Autodesk Inventor part; units mm, degrees
ref_plane "Work Plane1" through (0, 0, 39.4615) normal (0, 0, 1) x (1, 0, 0)
ref_plane "Work Plane2" through (-9.545, 0, 0) normal (1, 0, 0) x (0, 1, 0)
ref_plane "XZ Plane" through (0, 0, 0) normal (0, 1, 0) x (-1, 0, 0)
sketch "Sketch1" plane through (0, 0, 0) normal (0, 1, 0) x (-1, 0, 0)
  circle A0 centre (24.5999, -4.9022) radius 2.2225
  line L0 (26.4238, -3.6322) -> (26.6065, -3.6322)
  circle A1 centre (24.5999, 4.9022) radius 2.2225
  line L1 (26.6196, 9.4615) -> (23.1196, 9.4615)
  line L2 (26.6065, -9.4615) -> (20.6065, -9.4615)
  line L3 (26.4238, -6.1722) -> (26.6065, -6.1722)
  line L4 (23.1196, 9.4615) -> (23.1196, 14.4615)
  line L5 (-26.4238, -3.6322) -> (-26.6065, -3.6322)
  line L6 (-26.4238, -6.1722) -> (-26.6065, -6.1722)
  line L7 (-26.6065, -9.4615) -> (-20.6065, -9.4615)
  circle A2 centre (-24.5999, -4.9022) radius 2.2225
  circle A3 centre (-24.5999, 4.9022) radius 2.2225
  line L8 (-26.6196, 9.4615) -> (-23.1196, 9.4615)
  line L9 (-23.1196, 9.4615) -> (-23.1196, 14.4615)
  line L10 (20.6065, 10.9615) -> (-20.6065, 10.9615)
  line L11 (23.1196, 14.4615) -> (21.9202, 14.4615)
  line L12 (-12.375, 14.4615) -> (-23.1196, 14.4615)
  line L13 (21.9202, 14.4593) -> (21.9202, 39.4593)
  line L14 (21.9202, 14.4593) -> (46.9202, 14.4593) construction
  line L15 (21.9202, 39.4593) -> (-2.8298, 39.4615)
  line L16 (-2.8298, 39.4615) -> (-2.832, 14.4615)
  line L17 (-2.832, 14.4615) -> (-12.375, 14.4615)
  line L18 (-26.6196, 9.4615) -> (-29.5802, 9.4615)
  line L19 (-29.5802, 9.4615) -> (-29.5802, -9.4615)
  line L20 (-29.5802, -9.4615) -> (-26.6065, -9.4615)
  line L21 (26.6196, 9.4615) -> (29.5802, 9.4615)
  line L22 (29.5802, 9.4615) -> (29.5802, -9.4615)
  line L23 (29.5802, -9.4615) -> (26.6065, -9.4615)
  line L24 (-20.6065, -9.4615) -> (-20.6065, 10.9615)
  line L25 (20.6065, -9.4615) -> (20.6065, 10.9615)
  point P0 (-26.4238, 3.6322)
  point P1 (0, 0)
  point P2 (9.5452, 14.4593)
  dimension "d38" = 90
  dimension "d39" = 24.75
  dimension "d41" = 90
  dimension "d43" = 4.9803
  dimension "d45" = 4.9803
extrude "Extrusion1" add sketch "Sketch1" along normal blind 3 contours A0 | A1 | L21 L22 L23 L2 L25 L10 L24 L7 L20 L19 L18 L8 L9 L12 L17 L16 L15 L13 L11 L4 L1 | A2 | A3
ref_plane "Work Plane1" through (0, 0, 39.4615) normal (0, 0, 1) x (1, 0, 0)
sketch "Sketch2" plane through (0, 0, 39.4615) normal (0, 0, 1) x (1, 0, 0)
  circle A0 centre (-9.5452, 25) radius 9.125
  line L0 (-21.9202, 0) -> (2.8298, 0)
  arc A1 (2.8298, 25) -> (-21.9202, 25) centre (-9.5452, 25) ccw
  line L1 (2.8298, 0) -> (2.8298, 25)
  line L2 (-21.9202, 0) -> (-21.9202, 25)
  point P0 (0, 0)
  point P1 (-9.5452, 0)
  dimension "d23" = 18.25
  dimension "d24" = 24.75
  dimension "d25" = 24.75
  dimension "d26" = 25
  dimension "d27" = 25
extrude "Extrusion2" add sketch "Sketch2" along normal blind 3
extrude "Extrusion3" cut sketch "Sketch1" along normal up to next contours A0 | A1 | A2 | A3
sketch "Sketch3" plane through (0, 0, 0) normal (0, -1, 0) x (1, 0, 0)
  circle A0 centre (-24.5999, -4.9022) radius 2.2225
  circle A1 centre (-24.5999, 4.9022) radius 2.2225
  circle A2 centre (24.5999, 4.9022) radius 2.2225
  circle A3 centre (24.5999, -4.9022) radius 2.2225
  line L0 (-29.5802, -9.4615) -> (-20.6065, -9.4615)
  line L1 (-20.6065, -9.4615) -> (-20.6065, 10.9615)
  line L2 (-20.6065, 10.9615) -> (20.6065, 10.9615)
  line L3 (20.6065, 10.9615) -> (20.6065, -9.4615)
  line L4 (20.6065, -9.4615) -> (29.5802, -9.4615)
  line L5 (29.5802, -9.4615) -> (29.5802, 9.4615)
  line L6 (29.5802, 9.4615) -> (23.1196, 9.4615)
  line L7 (23.1196, 9.4615) -> (23.1196, 14.4615)
  line L8 (23.1196, 14.4615) -> (2.832, 14.4615)
  line L9 (2.832, 14.4615) -> (2.8298, 39.4615)
  line L10 (2.8298, 39.4615) -> (-21.9202, 39.4593)
  line L11 (-21.9202, 39.4593) -> (-21.9202, 14.4615)
  line L12 (-21.9202, 14.4615) -> (-23.1196, 14.4615)
  line L13 (-23.1196, 14.4615) -> (-23.1196, 9.4615)
  line L14 (-23.1196, 9.4615) -> (-29.5802, 9.4615)
  line L15 (-29.5802, 9.4615) -> (-29.5802, -9.4615)
  line L16 (-21.9202, 39.4615) -> (2.8298, 39.4615)
  line L17 (2.8298, 39.4615) -> (2.8298, 42.4615)
  line L18 (-21.9202, 42.4615) -> (2.8298, 42.4615)
  line L19 (-21.9202, 39.4615) -> (-21.9202, 42.4615)
  point P0 (0, 0)
extrude "Extrusion4" add sketch "Sketch3" along normal blind 2
sketch "Sketch4" plane through (0, -2, 0) normal (0, -1, 0) x (1, 0, 0)
  circle A0 centre (24.5999, -4.9022) radius 2.2225
  circle A1 centre (24.5999, 4.9022) radius 2.2225
  circle A2 centre (-24.5999, 4.9022) radius 2.2225
  circle A3 centre (-24.5999, -4.9022) radius 2.2225
  line L0 (-29.5802, -9.4615) -> (-20.6065, -9.4615)
  line L1 (-20.6065, -9.4615) -> (-20.6065, 10.9615)
  line L2 (-20.6065, 10.9615) -> (20.6065, 10.9615)
  line L3 (20.6065, 10.9615) -> (20.6065, -9.4615)
  line L4 (20.6065, -9.4615) -> (29.5802, -9.4615)
  line L5 (29.5802, -9.4615) -> (29.5802, 9.4615)
  line L6 (29.5802, 9.4615) -> (23.1196, 9.4615)
  line L7 (23.1196, 9.4615) -> (23.1196, 14.4615)
  line L8 (23.1196, 14.4615) -> (2.832, 14.4615)
  line L9 (2.832, 14.4615) -> (2.8298, 39.4615)
  line L10 (2.8298, 39.4615) -> (-21.9202, 39.4593)
  line L11 (-21.9202, 39.4593) -> (-21.9202, 14.4615)
  line L12 (-21.9202, 14.4615) -> (-23.1196, 14.4615)
  line L13 (-23.1196, 14.4615) -> (-23.1196, 9.4615)
  line L14 (-23.1196, 9.4615) -> (-29.5802, 9.4615)
  line L15 (-29.5802, 9.4615) -> (-29.5802, -9.4615)
  line L16 (2.832, 14.4615) -> (23.1196, 14.4615)
  line L17 (23.1196, 14.4615) -> (23.1196, 16.4615)
  line L18 (23.1196, 16.4615) -> (2.832, 16.4615)
  line L19 (2.832, 16.4615) -> (2.832, 14.4615)
  line L20 (-21.9202, 14.4615) -> (-23.1196, 14.4615)
  line L21 (-23.1196, 14.4615) -> (-23.1196, 16.4615)
  line L22 (-23.1196, 16.4615) -> (-21.9202, 16.4615)
  line L23 (-21.9202, 16.4615) -> (-21.9202, 14.4615)
  point P0 (0, 0)
  dimension "d52" = 2
  dimension "d53" = 2
extrude "Extrusion5" add sketch "Sketch4" against normal blind 5 contours L21 L22 L11 L12 | L8 L9 L18 L17
sketch "Sketch5" plane through (0, -2, 0) normal (0, -1, 0) x (1, 0, 0)
  line L0 (20.6065, 10.9615) -> (-20.6065, 10.9615)
  line L1 (-20.6065, 10.9615) -> (-20.6065, 11.9615)
  line L2 (-20.6065, 11.9615) -> (20.6065, 11.9615)
  line L3 (20.6065, 11.9615) -> (20.6065, 10.9615)
  point P0 (0, 0)
  dimension "d56" = 1
extrude "Extrusion6" cut sketch "Sketch5" against normal up to next
sketch "Sketch6" plane through (0, -2, 0) normal (0, -1, 0) x (1, 0, 0)
  line L0 (21.6065, 11.9615) -> (-21.6065, 11.9615)
  line L1 (-21.6065, 11.9615) -> (-21.6065, -9.4615)
  line L2 (-21.6065, -9.4615) -> (21.6065, -9.4615)
  line L3 (21.6065, -9.4615) -> (21.6065, 11.9615)
  line L4 (20.6065, 11.9615) -> (20.6065, -9.4615)
  line L5 (-20.6065, -9.4615) -> (-20.6065, 11.9615)
  line L6 (-20.6065, 11.9615) -> (20.6065, 11.9615)
  point P0 (0, 0)
  dimension "d59" = 1
  dimension "d60" = 1
  dimension "d61" = 0
extrude "Extrusion7" cut sketch "Sketch6" against normal up to next
sketch "Sketch7" plane through (0, -2, 0) normal (0, -1, 0) x (1, 0, 0)
  line L0 (-23.1196, 9.4615) -> (-29.5802, 9.4615)
  line L1 (-29.5802, 9.4615) -> (-29.5802, 16.4615)
  line L2 (-29.5802, 16.4615) -> (-23.1196, 16.4615)
  line L3 (-23.1196, 16.4615) -> (-23.1196, 9.4615)
  line L4 (23.1196, 9.4615) -> (29.5802, 9.4615)
  line L5 (29.5802, 9.4615) -> (29.5802, 16.4615)
  line L6 (29.5802, 16.4615) -> (23.1196, 16.4615)
  line L7 (23.1196, 16.4615) -> (23.1196, 9.4615)
  point P0 (0, 0)
  dimension "d64" = 7
  dimension "d65" = 6.4606
extrude "Extrusion8" add sketch "Sketch7" against normal blind 5
sketch "Sketch8" plane through (0, -2, 0) normal (0, -1, 0) x (1, 0, 0)
  line L0 (-29.5802, -9.4615) -> (-21.6062, -9.4615)
  line L1 (-21.6062, -9.4615) -> (-21.6062, -14.4615)
  line L2 (-21.6062, -14.4615) -> (-29.5802, -14.4615)
  line L3 (-29.5802, -14.4615) -> (-29.5802, -9.4615)
  point P0 (0, 0)
  dimension "d68" = 7.974
  dimension "d69" = 5
extrude "Extrusion9" add sketch "Sketch8" against normal blind 5
mirror "Mirror1" about plane through (0, 0, 0) normal (1, 0, 0) of "Extrusion9"
sketch "Sketch9" plane through (0, -2, 0) normal (0, -1, 0) x (1, 0, 0)
  line L0 (-29.5802, -14.4615) -> (-29.5802, 16.4615)
  line L1 (-29.5802, 12) -> (29.5798, 12)
  line L2 (29.5798, 12) -> (29.5798, 19)
  line L3 (29.5798, 19) -> (-29.5802, 19)
  line L4 (-29.5802, 19) -> (-29.5802, 12)
  point P0 (0, 0)
  dimension "d72" = 59.16
extrude "Extrusion10" add sketch "Sketch9" against normal blind 5
sketch "Sketch10" plane through (0, 0, 42.4615) normal (0, 0, 1) x (1, 0, 0)
  circle A0 centre (-9.5452, 25) radius 9.125
  line L0 (2.8298, 0) -> (2.8298, 25)
  arc A1 (2.8298, 25) -> (-21.9202, 25) centre (-9.5452, 25) ccw
  line L1 (-21.9202, 25) -> (-21.9202, -2)
  line L2 (2.8298, -2) -> (-21.9202, -2)
  line L3 (2.8298, 0) -> (2.8298, -2)
  point P0 (0, 0)
extrude "Extrusion11" add sketch "Sketch10" along normal blind 2
ref_plane "Work Plane2" through (-9.545, 0, 0) normal (1, 0, 0) x (0, 1, 0)
sketch "Sketch12" plane through (-9.545, 0, 0) normal (1, 0, 0) x (0, 1, 0)
  line L0 (3, 39.4615) -> (8, 39.4615)
  line L1 (8, 39.4615) -> (3, 34.4615)
  line L2 (3, 34.4615) -> (3, 39.4615)
  line L3 (3, 39.4615) -> (8, 39.4615)
  line L4 (3, 39.4615) -> (25, 39.4615)
  point P0 (0, 0)
  dimension "d79" = 5
  dimension "d80" = 45
  dimension "d83" = 5
extrude "Extrusion12" add sketch "Sketch12" along normal mid plane 24.75
equation "\"d45\" = d44"
equation "\"d27\" = d26"
properties part number "Dudukan Proximity Servo"
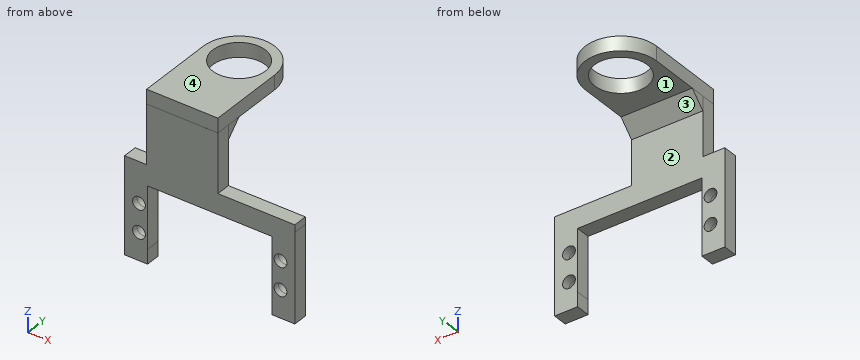
Could you check a few things on this model? Use its own coordinates, in mm. Face numbers are marked on the shaded views. Give positions to 0.01 mm unless a question says otherwise; leave off trailing zeros. Order: outer loops, then holes, each group sorted by start corner. A loop starts at its lowest first (then second) coordinate and runs counter-clockwise, first axis right, second up.
1. Suppose I cut it at D-D (x = 23.5). List the corners of the cut face in (y, z) for me.
2. We'd pull the mould along Z, two halves only. Please class the marked faces 1, 2, 3 and 4: pulls with the +Z half, pulls with the -Z half, needs draft (parallel to the pull), parting line crosses it, or undercut.
3. Suppose I cut it at A-A (z = 10). List the corners of the cut face in (x, y) for me, plus the area to 3 significant figures.
4. Will these pins go through, and if not, where does the flat tip stop? P1, Ø5.5, axis at y = 6.5, z = 36.5, coming from the +X side; P2, Ø5.5, axis at x = 9.5, y = 0.5, coming from the +Z side; P3, Ø6, axis at x = -24.6, z = 4.9, coming from the -Y side; P4, Ø10, axis at x = 6.5, y = 9, coming from the -Z side.
5. I need wall thicknesses on L1, parallel to X at y = 4, z = 39; L2, parallel to Z at x = -8, y = 13; L3, parallel to Y at x = -13.5, z = 19. Which ranges of each line are inside material? Lowest first, please.
6. Suppose I cut it at B-B (y = 27.5). List the corners of the cut face in (x, z) for me.
Solved:
1. outline: (-2, -14.46) - (3, -14.46) - (3, -6.83) - (-2, -6.83) - close; (-2, -2.97) - (3, -2.97) - (3, 2.97) - (-2, 2.97) - close; (-2, 6.83) - (3, 6.83) - (3, 19) - (-2, 19) - close
2. face 1: undercut
2. face 2: needs draft
2. face 3: pulls with the -Z half
2. face 4: pulls with the +Z half
3. outline: (-29.58, -2) - (-21.61, -2) - (-21.61, 3) - (-29.58, 3) - close; (21.61, -2) - (29.58, -2) - (29.58, 3) - (21.61, 3) - close
3. area: 79.7 mm2
4. P1: stops at x = 2.83
4. P2: stops at z = 19
4. P3: stops at y = -2
4. P4: stops at z = 37.07
5. L1: x = -21.92 to 2.83
5. L2: z = 39.46 to 44.46
5. L3: y = -2 to 3
6. outline: (-21.67, 39.46) - (-18.32, 39.46) - (-18.32, 44.46) - (-21.67, 44.46) - close; (-0.77, 39.46) - (2.57, 39.46) - (2.57, 44.46) - (-0.77, 44.46) - close
